from build123d import *

# Parameters (mm, degrees)
F0_W      = 25
F0_H      = 25
F1_DEPTH  = 40
F2_W      = 21
F2_H      = 80
F3_DEPTH  = 1.5
F4_W      = 21
F4_H      = 80
F5_DEPTH  = 1.5
F7_DEPTH  = 21
F9_DEPTH  = 4
F10_R     = 2.5
F11_DEPTH = 4.001
F13_DEPTH = 4


with BuildPart() as f1:
    # F0 (on Front) → F1 (new body, symmetric)
    with BuildSketch(Plane.XZ):
        Rectangle(F0_W, F0_H)
    extrude(amount=F1_DEPTH, both=True)

    # F2 (on face) → F3 (cut)
    with BuildSketch(Plane.XY.offset(12.5)):
        with Locations((-2, 0)):
            Rectangle(F2_W, F2_H)
    extrude(amount=-F3_DEPTH, mode=Mode.SUBTRACT)

    # F4 (on face) → F5 (cut)
    with BuildSketch(Plane(origin=(0, 0, -12.5), x_dir=(1, 0, 0), z_dir=(0, 0, -1))):
        with Locations((-2, 0)):
            Rectangle(F4_W, F4_H)
    extrude(amount=-F5_DEPTH, mode=Mode.SUBTRACT)

    # F6 (on face) → F7 (cut)
    with BuildSketch(Plane(origin=(-12.5, 0, 0), x_dir=(0, -1, 0), z_dir=(-1, 0, 0))):
        with BuildLine():
            Line((-40, 11), (-40, -11))
            ThreePointArc((-40, -11), (-29, 0), (-40, 11))
        make_face()
    extrude(amount=-F7_DEPTH, mode=Mode.SUBTRACT)

    # F8 (on face) → F9 (join)
    with BuildSketch(Plane(origin=(8.5, 0, 0), x_dir=(0, -1, 0), z_dir=(-1, 0, 0))):
        with BuildLine():
            Line((-40, -11), (-40, 11))
            ThreePointArc((-40, 11), (-51, 0), (-40, -11))
        make_face()
    extrude(amount=-F9_DEPTH)

    # F10 (on face) → F11 (cut, through all)
    with BuildSketch(Plane(origin=(8.5, 0, 0), x_dir=(0, -1, 0), z_dir=(-1, 0, 0))):
        with Locations((-40, 0)):
            Circle(F10_R)
    extrude(amount=-F11_DEPTH, mode=Mode.SUBTRACT)

    # F12 (on face) → F13 (join)
    with BuildSketch(Plane.YZ.offset(12.5)):
        with BuildLine():
            ThreePointArc((48.771264901, 6.6381407063), (48.1972510553, 7.3351942808), (47.5679988761, 7.9828186132))
            add(Edge.make_bspline(
                [(47.5679988761, 7.9828186132), (48.3027333045, 7.2337960601), (48.7357424374, 6.6842950025), (48.771264901, 6.6381407063)],
                knots=[7.1076445711, 7.1076445711, 7.1076445711, 7.1076445711, 10.5497147991, 10.5497147991, 10.5497147991, 10.5497147991], degree=3))
        make_face()
        with BuildLine():
            add(Edge.make_bspline(
                [(40, 12.5), (43.2471029485, 11.9269308431), (46.0508214725, 9.5295000376), (47.5679988761, 7.9828186132)],
                knots=[0, 0, 0, 0, 7.1076445711, 7.1076445711, 7.1076445711, 7.1076445711], degree=3))
            Line((40, 12.5), (40, 11))
            ThreePointArc((40, 11), (44.0736344494, 10.2179010747), (47.5679988761, 7.9828186132))
        make_face()
        with BuildLine():
            add(Edge.make_bspline(
                [(47.5679988761, -7.9828186132), (48.3027333045, -7.2337960601), (48.7357424374, -6.6842950025), (48.771264901, -6.6381407063)],
                knots=[7.1076445711, 7.1076445711, 7.1076445711, 7.1076445711, 10.5497147991, 10.5497147991, 10.5497147991, 10.5497147991], degree=3))
            ThreePointArc((47.5679988761, -7.9828186132), (48.1972510553, -7.3351942808), (48.771264901, -6.6381407063))
        make_face()
        with BuildLine():
            Line((40, -11), (40, -12.5))
            add(Edge.make_bspline(
                [(40, -12.5), (43.2471029485, -11.9269308431), (46.0508214725, -9.5295000376), (47.5679988761, -7.9828186132)],
                knots=[0, 0, 0, 0, 7.1076445711, 7.1076445711, 7.1076445711, 7.1076445711], degree=3))
            ThreePointArc((47.5679988761, -7.9828186132), (44.0736344494, -10.2179010747), (40, -11))
        make_face()
    extrude(amount=-F13_DEPTH)


solid = f1.part
Verification items for the finished model (mm, model axes). A direction names the side the tool comes from. Give positions to 0.01 mm unless a question says otherwise; leave off trailing zeros. Write each loop counter-clockwise with the first axis right and the second up, starting at its lowest first coordinate (ties: lowest second). Pieces come first, ordered by that corner, then holes.
(1) Cross-section at B-B (y = -7.5). Enter the section's corners in (x, z), plus the area to 3 significant figures.
(2) Mould release check, pull along Z, two halves, no side actions. Record for faces 4 (the face through (-2, 1, 11)), 5 (the face through (10, 51, 0)), 6 (the face through (10.47, 37.69, -0.96)), 7 (the face through (12.5, 6, 0)): +Z half, -Z half, draft (parallel to the pull), parting line (faces both ways), or undercut.
(3) Access from +Z, -Z, +X, -X, +Y, -Y to the whole of each face (thin tool, end or side, straight path). Record for faces 1 (the face through (-2, 29, 0)), 2 (the face through (-2, -1, -11)), 3 (the face through (0, -40, 0)).
(4) Material ranges on line 1 (Z direction, x = 10.7, y = 40); line 2 (X direction, y = 41, z = -8.25); line 3 (Z direction, x = -6.5, y = -16.5), recorded low to high.
(5) Cross-section at C-C (x = -4.5). Enter the section's corners in (y, z), plus the area to 3 significant figures.
(6) Gauge pin test, flat ends, axial feed: pin 1 (2 mm diameter, centred on y = 40.5, z = -4.5, fed in from -X); pin 2 (10 mm diameter, centred on x = -9.5, z = 4.5, fed in from +Y); pin 3 (6 mm diameter, centred on x = 5, y = -1, fed in from +Z). Record the tip position at first contact, or that the pin passes through.
(7) Cross-section at A-A (z = 0). Enter the section's corners in (x, y).
Worked out:
1. outline: (-12.5, -11) - (8.5, -11) - (8.5, -12.5) - (12.5, -12.5) - (12.5, 12.5) - (8.5, 12.5) - (8.5, 11) - (-12.5, 11) - close
1. area: 562 mm2
2. face 4: +Z half
2. face 5: parting line
2. face 6: undercut
2. face 7: draft
3. face 1: -X, +Y
3. face 2: -Z, -X, +Y, -Y
3. face 3: +Z, -Z, +X, -X, -Y
4. line 1: z = -12.5 to -2.5, 2.5 to 12.5
4. line 2: x = 8.5 to 12.5
4. line 3: z = -11 to 11
5. outline: (-40, -11) - (40, -11) arc R11 cw to (40, 11) - (-40, 11) - close
5. area: 1,570 mm2
6. pin 1: stops at x = 8.5
6. pin 2: stops at y = 34.45
6. pin 3: stops at z = 11
7. outline: (-12.5, -40) - (12.5, -40) - (12.5, 37.5) - (8.5, 37.5) - (8.5, 29) - (-12.5, 29) - close; (8.5, 42.5) - (12.5, 42.5) - (12.5, 51) - (8.5, 51) - close
